Model file for the job. Use its own axes, mm. Coordinates: 2 decimals unless noted, no trailing zeros. Write each loop counter-clockwise with the first axis right and the second up, starting at its lowest first coordinate (ties: lowest second). Pieces come first, ordered by that corner, then holes. Notation, with made-up numbers: (67.5, 84) -> (86.5, 84) arc R28 ccw to (86.5, 119) -> close; hole circle Ø3 at (69, -8.75). An arc over 180 degrees is marked (long way). Write item = value, one per line. Start each with the question number.
from build123d import *

# Parameters (mm, degrees)
SKETCH1_W           = 50
SKETCH1_H           = 1200
BOSS_EXTRUDE1_DEPTH = 150
CUT_EXTRUDE4_DEPTH  = 1216.781641579
SKETCH18_W          = 5
SKETCH18_H          = 140
CUT_EXTRUDE6_DEPTH  = 944.345111823
SKETCH19_W          = 5
SKETCH19_H          = 140
CUT_EXTRUDE7_DEPTH  = 944.345111823
SKETCH20_R          = 10
CUT_EXTRUDE8_DEPTH  = 944.345111823


with BuildPart() as part:
    # Sketch1 → Boss-Extrude1 (new body)
    with BuildSketch(Plane(origin=(0, 0, 0), x_dir=(1, 0, 0), z_dir=(0, 1, 0))):
        with Locations((-100, 330)):
            Rectangle(SKETCH1_W, SKETCH1_H)
    extrude(amount=BOSS_EXTRUDE1_DEPTH)

    # Sketch16 → Cut-Extrude4 (cut, through all)
    with BuildSketch(Plane.XY.offset(270)):
        Polygon((-100, 5), (-120, 5), (-120, 145), (-80, 145), (-80, 5), align=None)
    extrude(amount=-CUT_EXTRUDE4_DEPTH, mode=Mode.SUBTRACT)

    # Sketch18 → Cut-Extrude6 (cut, through all)
    with BuildSketch(Plane(origin=(-75, 0, 0), x_dir=(0, 0, -1), z_dir=(1, 0, 0))):
        with Locations((-247.5, 75)):
            Rectangle(SKETCH18_W, SKETCH18_H)
    extrude(amount=-CUT_EXTRUDE6_DEPTH, mode=Mode.SUBTRACT)

    # Sketch19 → Cut-Extrude7 (cut, through all)
    with BuildSketch(Plane(origin=(-75, 0, 0), x_dir=(0, 0, -1), z_dir=(1, 0, 0))):
        with Locations((-202.5, 75)):
            Rectangle(SKETCH19_W, SKETCH19_H)
    extrude(amount=-CUT_EXTRUDE7_DEPTH, mode=Mode.SUBTRACT)

    # Sketch20 → Cut-Extrude8 (cut, through all)
    with BuildSketch(Plane(origin=(-75, 0, 0), x_dir=(0, 0, -1), z_dir=(1, 0, 0))):
        with Locations((-130, 75)):
            Circle(SKETCH20_R)
        with Locations((850, 75)):
            Circle(SKETCH20_R)
    extrude(amount=-CUT_EXTRUDE8_DEPTH, mode=Mode.SUBTRACT)


solid = part.part
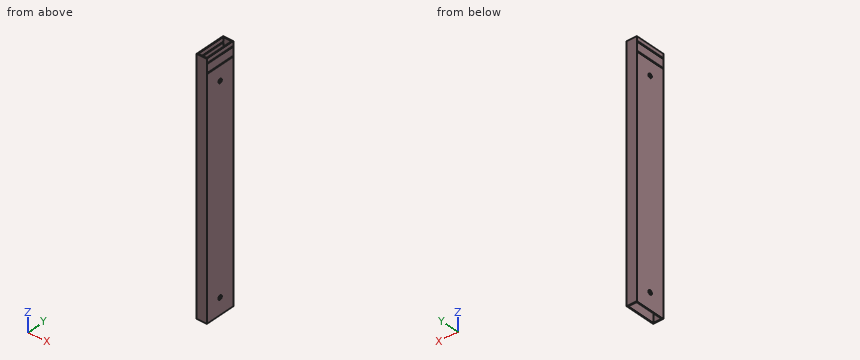
(1) Saw through at D-D (z = -850). Give the cut face in (x, y).
(2) Saw through at C-C (x = -95.5). Give the cut face in (y, z).
(3) Drop a flat-ended pin along its axis: pin 1 Ø12 at (x, z) = (-85, -26) entering from -Y. Give the stop position or say it passes through.
(4) Saw through at A-A (y = 23). Give the cut face in (x, z), then the cut area to 3 significant figures.
(5) Drill centre lines: line 1 along X through (y, z) = (82.5, -569.5); line 2 along Y through (x, z) = (-78, -850); line 3 along Y through (x, z) = (-86, -734). Where is each one in solid material? Low to high.
(6) Saw through at B-B (z = -653). Give the cut face in (x, y), then the cut area to 3 significant figures.
Returned:
q1.outline = (-125, 0) -> (-75, 0) -> (-75, 65) -> (-80, 65) -> (-80, 5) -> (-120, 5) -> (-120, 65) -> (-125, 65) -> close; (-125, 85) -> (-120, 85) -> (-120, 145) -> (-80, 145) -> (-80, 85) -> (-75, 85) -> (-75, 150) -> (-125, 150) -> close
q2.outline = (0, -930) -> (5, -930) -> (5, 270) -> (0, 270) -> close; (145, -930) -> (150, -930) -> (150, 270) -> (145, 270) -> close
q3.pin_1 = 0
q4.outline = (-125, -930) -> (-120, -930) -> (-120, 200) -> (-125, 200) -> close; (-125, 205) -> (-120, 205) -> (-120, 245) -> (-125, 245) -> close; (-125, 250) -> (-120, 250) -> (-120, 270) -> (-125, 270) -> close; (-80, -930) -> (-75, -930) -> (-75, 200) -> (-80, 200) -> close; (-80, 205) -> (-75, 205) -> (-75, 245) -> (-80, 245) -> close; (-80, 250) -> (-75, 250) -> (-75, 270) -> (-80, 270) -> close
q4.area = 11,900 mm2
q5.line_1 = -125 to -120, -80 to -75
q5.line_2 = 0 to 65, 85 to 150
q5.line_3 = 0 to 5, 145 to 150
q6.outline = (-125, 0) -> (-75, 0) -> (-75, 150) -> (-125, 150) -> close; hole (-120, 5) -> (-80, 5) -> (-80, 145) -> (-120, 145) -> close
q6.area = 1,900 mm2
